Geometry check sheet. Reference: the model listing, model coordinates, mm. Coordinates: 2 decimals unless noted, no trailing zeros. Loops run counter-clockwise (first coordinate to the right, second up) from the corner with the lowest first, then second, coordinate; pieces in that order, holes last. Notation, with made-up numbers: M 29.25,34 L 80.25,34 A24 cw 80.25,62 Z; hole C 23.5,-3.75 d10. An arc over 180 degrees is marked long. Use CSV: the item, a comma, the result in double quotes.
```python
from build123d import *

# Parameters (mm, degrees)
F0_W     = 69.189604
F0_H     = 67.970401
F1_DEPTH = 46.99
F4_D     = 25.4
F5_D     = 6.35
F6_D     = 6.35


with BuildPart() as f1:
    # F0 (on Front) → F1 (new body)
    with BuildSketch(Plane.XZ):
        with Locations((1.2192, 2.895598)):
            Rectangle(F0_W, F0_H)
    extrude(amount=F1_DEPTH)

    # F4 (through all)
    with Locations(Plane(origin=(0, 0, 0), x_dir=(-1, 0, 0), z_dir=(0, 1, 0))):
        with Locations((0, 6.492837)):
            Hole(F4_D / 2)

    # F5 (through all)
    with Locations(Plane(origin=(0, 0, 0), x_dir=(-1, 0, 0), z_dir=(0, 1, 0))):
        with Locations((-20.368258, 21.817673)):
            Hole(F5_D / 2)

    # F6 (through all)
    with Locations(Plane(origin=(0, 0, 0), x_dir=(-1, 0, 0), z_dir=(0, 1, 0))):
        with Locations((16.558066, 19.802285)):
            Hole(F6_D / 2)


solid = f1.part
```
1. Thickness scan on line 1 (Z direction, x = 0, y = -29); line 2 (X direction, y = -23.5, z = 21); line 3 (X direction, y = -25.5, z = 13). Record the ranges inside material, lowest first. Write a range as [from, to].
The answers:
line 1,"[-31.09, -6.21], [19.19, 36.88]"
line 2,"[-33.38, -19.5], [-13.62, 17.3], [23.44, 35.81]"
line 3,"[-33.38, -10.91], [10.91, 35.81]"
2. Section check A-A, the plane x = 0. Record the cut outline in (y, z), plus the area to 3 significant figures.
The answers:
outline,"M -46.99,-31.09 L 0,-31.09 L 0,-6.21 L -46.99,-6.21 Z; M -46.99,19.19 L 0,19.19 L 0,36.88 L -46.99,36.88 Z"
area,"2,000 mm^2"
3. Section check B-B, the plane z = -3.5. Record the cut outline in (x, y), plus the area to 3 significant figures.
The answers:
outline,"M -33.38,-46.99 L -7.84,-46.99 L -7.84,0 L -33.38,0 Z; M 7.84,-46.99 L 35.81,-46.99 L 35.81,0 L 7.84,0 Z"
area,"2,510 mm^2"
4. Gauge pin test, flat end, axial feed: P1, Ø15, axis at x = 0, z = 6.49, coming from the -Y side. Record the tip position at first contact, or that the pin passes through.
The answers:
P1,"through"
5. Section check C-C, the plane y = -21. Record the cut outline in (x, z) (3 decimals).
The answers:
outline,"M -33.376,-31.09 L 35.814,-31.09 L 35.814,36.881 L -33.376,36.881 Z; hole C -16.558,19.802 d6.35; hole C 0,6.493 d25.4; hole C 20.368,21.818 d6.35"
6. Release check for a two-part mould opening along X. For faces 1 (the flat face through (-33.376, -23, 2)), 2 (the cylindrical face through (-17.246, -23.824, 16.703)), 3 (the flat face through (8, 0, -4)) record: +X half, -X half, draft (parallel to the pull), parting line (faces both ways), or undercut.
The answers:
face 1,"-X half"
face 2,"undercut"
face 3,"draft"
